```python
from build123d import *

# Parameters (mm, degrees)
SKETCH1_R           = 1.5
BOSS_EXTRUDE1_DEPTH = 4


with BuildPart() as part:
    # Sketch1 → Boss-Extrude1 (new body)
    with BuildSketch(Plane(origin=(0, 0, 0), x_dir=(1, 0, 0), z_dir=(0, 1, 0))):
        with BuildLine():
            ThreePointArc((-5.489268293, 0.343414634), (0, -5.5), (5.489268293, 0.343414634))
            ThreePointArc((5.489268293, 0.343414634), (4.25, 40), (5.489268293, 79.656585366))
            ThreePointArc((5.489268293, 79.656585366), (0, 85.5), (-5.489268293, 79.656585366))
            ThreePointArc((-5.489268293, 79.656585366), (-4.25, 40), (-5.489268293, 0.343414634))
        make_face()
        Circle(SKETCH1_R, mode=Mode.SUBTRACT)
        with Locations((0, 80)):
            Circle(SKETCH1_R, mode=Mode.SUBTRACT)
        with Locations((0, 40)):
            Circle(SKETCH1_R, mode=Mode.SUBTRACT)
    extrude(amount=BOSS_EXTRUDE1_DEPTH)


solid = part.part
```
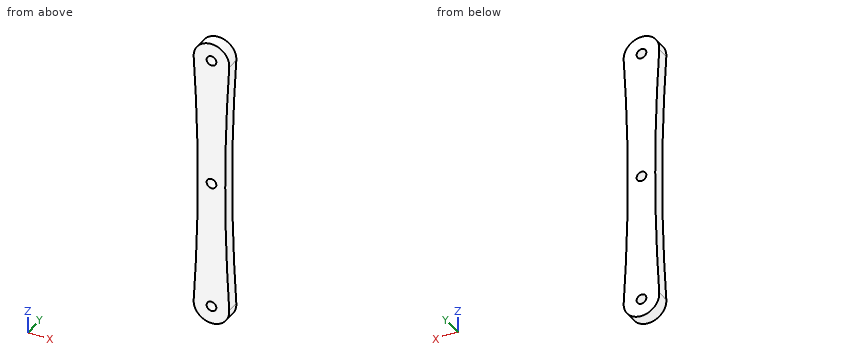
Can you work these out from the model? Positions are in its coordinate system, mm. Coordinates: 2 decimals unless noted, no trailing zeros. Order: outer loops, then holes, each group sorted by start corner. A loop starts at its lowest first (then second) coordinate and runs counter-clockwise, first axis right, second up. Notation, with made-up numbers: (22.5, -6.75) -> (54.5, -6.75) arc R21 cw to (54.5, 25.25) -> close; hole circle Ø3 at (11.25, 57.5). An arc over 180 degrees is marked (long way). Write each question's results on one line, items separated by ' | '.
Item 1: I want a section at D-D, the plane z = -5.5. Write out the boundary of the cut face in (x, y), then the cut area to 3 significant figures.
Results are:
outline: (-5.19, 0) -> (5.19, 0) -> (5.19, 4) -> (-5.19, 4) -> close | area: 41.5 mm²
Item 2: If I drill on line 1 along Z through (x, y) = (0, 2.8); line 2 along X through (y, z) = (1.55, -40); line 3 along X through (y, z) = (0.95, -80), over which ranges is the centre line in solid material (lowest first)?
Results are:
line 1: -85.5 to -81.5, -78.5 to -41.5, -38.5 to -1.5, 1.5 to 5.5 | line 2: -4.25 to -1.5, 1.5 to 4.25 | line 3: -5.5 to -1.5, 1.5 to 5.5
Item 3: I want a section at B-B, the plane y = 2.4. Write out the boundary of the cut face in (x, z) (3 decimals), then the cut area to 3 significant figures.
Results are:
outline: (-5.489, -79.657) arc R5.5 ccw (long way) to (5.489, -79.657) arc R635.125 cw to (5.489, -0.343) arc R5.5 ccw (long way) to (-5.489, -0.343) arc R635.125 cw to start; hole circle Ø3 at (0, -80); hole circle Ø3 at (0, -40); hole circle Ø3 at (0, 0) | area: 821 mm²
Item 4: I want a section at A-A, the plane x = 0. Write out the boundary of the cut face in (y, z), then the cut area to 3 significant figures.
Results are:
outline: (0, -85.5) -> (4, -85.5) -> (4, -81.5) -> (0, -81.5) -> close; (0, -78.5) -> (4, -78.5) -> (4, -41.5) -> (0, -41.5) -> close; (0, -38.5) -> (4, -38.5) -> (4, -1.5) -> (0, -1.5) -> close; (0, 1.5) -> (4, 1.5) -> (4, 5.5) -> (0, 5.5) -> close | area: 328 mm²
Item 5: I want a section at C-C, the plane z = -40. Write out the boundary of the cut face in (x, y).
Results are:
outline: (-4.25, 0) -> (-1.5, 0) -> (-1.5, 4) -> (-4.25, 4) -> close; (1.5, 0) -> (4.25, 0) -> (4.25, 4) -> (1.5, 4) -> close
